Model file for the job. Use its own axes, mm. A direction names the side the tool comes from. Give positions to 0.01 mm unless a question says otherwise; leave off trailing zeros. Write each loop counter-clockwise with the first axis right and the second up, starting at its lowest first coordinate (ties: lowest second). Pieces come first, ordered by that corner, then holes. Notation, with made-up numbers: (58.25, 64) - (62.25, 64) arc R29 ccw to (62.25, 87) - close; hole circle Ø9 at (41.5, 72). An arc over 180 degrees is marked (long way). One line per item, written item: value. Start each with the question number.
(1) Cut at D-D, the plane x = -23. List the corners of the cut face in (y, z).
(2) Cut at A-A, the plane x = 0. List the corners of the cut face in (y, z), and give its area (3 significant figures).
(3) Drop flat-ended pins along their axis: P1, Ø8, axis at y = -27.5, z = 14.5, coming from the -X side; P2, Ø1.5, axis at y = 27.5, z = 11.5, coming from the -X side; P3, Ø8, axis at x = 12, z = 7.5, coming from the -Y side. Give the stop position or say it passes through.
(4) Cut at C-C, the plane y = 63.5. List the corners of the cut face in (x, z), and give its area (3 significant figures).
(5) Cut at B-B, the plane y = 0. List the corners of the cut face in (x, z).
(6) Mould opens along Y. For faces 6 (the face through (-35.2, -72.74, 12.52)), 7 (the face through (25.17, 51.98, 12.52)), 8 (the face through (-19, 3, 25.4)), 9 (the face through (-56.276, 12.977, 12.522)) say: pulls with the +Y half, pulls with the -Y half, needs draft (parallel to the pull), parting line crosses it, or undercut.
(7) Probe L1, parallel to Y at x = 0, z = 10.5; L2, parallel to X at y = 56, z = 14; L3, parallel to X at y = -58, z = 14. List the from-to ranges inside material, lowest first.
(8) 3-axis set-ups, long thin cutter, end or side, ignore diameter. For faces 1 (the face through (-45.39, 53.94, 12.52)), 2 (the face through (70.77, -2, 12.52)), 3 (the face through (17.49, -68.29, 12.52)), 4 (the face through (-42.49, -56.26, 12.52)), 5 (the face through (34.922, -72.876, 12.522)): which of +Z, -Z, +X, -X, +Y, -Y reach the whole face in a straight line?
from build123d import *

# Parameters (mm, degrees)
F0_R     = 19.05
F1_DEPTH = 25.4


with BuildPart() as f1:
    # F0 (on Top) → F1 (new body)
    with BuildSketch(Plane.XY):
        with BuildLine():
            Line((-10.182837, -59.196547), (-9.157953, -57.02169))
            ThreePointArc((-9.157953, -57.02169), (-25.057833, -52.033126), (-38.871462, -42.712418))
            Line((-38.871462, -42.712418), (-39.932829, -44.869706))
            Line((-39.932829, -44.869706), (-45.115972, -67.966514))
            Line((-45.115972, -67.966514), (-35.062492, -72.808015))
            Line((-35.062492, -72.808015), (-25.009012, -77.649516))
            Line((-25.009012, -77.649516), (-10.182837, -59.196547))
        make_face()
        with BuildLine():
            Line((-52.630619, -28.947181), (-50.291243, -28.392466))
            ThreePointArc((-50.291243, -28.392466), (-56.30444, -12.851121), (-57.629873, 3.760176))
            Line((-57.629873, 3.760176), (-59.97826, 3.244939))
            Line((-59.97826, 3.244939), (-81.267709, -7.103341))
            Line((-81.267709, -7.103341), (-78.784705, -17.982095))
            Line((-78.784705, -17.982095), (-76.3017, -28.860849))
            Line((-76.3017, -28.860849), (-52.630619, -28.947181))
        make_face()
        with BuildLine():
            ThreePointArc((-53.554201, 21.616864), (-45.152655, 36.008041), (-32.991815, 47.401281))
            Line((-32.991815, 47.401281), (-34.858838, 48.916078))
            Line((-34.858838, 48.916078), (-56.223203, 59.108793))
            Line((-56.223203, 59.108793), (-63.180428, 50.38471))
            Line((-63.180428, 50.38471), (-70.137652, 41.660627))
            Line((-70.137652, 41.660627), (-55.446471, 23.100003))
            Line((-55.446471, 23.100003), (-53.554201, 21.616864))
        make_face()
        with BuildLine():
            ThreePointArc((32.991815, 47.401281), (45.152655, 36.008041), (53.554201, 21.616864))
            Line((53.554201, 21.616864), (55.446471, 23.100003))
            Line((55.446471, 23.100003), (70.137652, 41.660627))
            Line((70.137652, 41.660627), (63.180428, 50.38471))
            Line((63.180428, 50.38471), (56.223203, 59.108793))
            Line((56.223203, 59.108793), (34.858838, 48.916078))
            Line((34.858838, 48.916078), (32.991815, 47.401281))
        make_face()
        with BuildLine():
            ThreePointArc((0, 57.752413), (8.332046, 57.148213), (16.489754, 55.348254))
            Line((16.489754, 55.348254), (16.51, 57.752413))
            Line((16.51, 57.752413), (11.158521, 80.8108))
            Line((11.158521, 80.8108), (0, 80.8108))
            Line((0, 80.8108), (0, 57.752413))
        make_face()
        with BuildLine():
            ThreePointArc((-16.489754, 55.348254), (-8.332046, 57.148213), (0, 57.752413))
            Line((0, 57.752413), (0, 80.8108))
            Line((0, 80.8108), (-11.158521, 80.8108))
            Line((-11.158521, 80.8108), (-16.51, 57.752413))
            Line((-16.51, 57.752413), (-16.489754, 55.348254))
        make_face()
        with BuildLine():
            ThreePointArc((57.629873, 3.760176), (57.72177, 1.881086), (57.752413, 0))
            ThreePointArc((57.752413, 0), (55.855984, -14.678225), (50.291243, -28.392466))
            Line((50.291243, -28.392466), (52.630619, -28.947181))
            Line((52.630619, -28.947181), (76.3017, -28.860849))
            Line((76.3017, -28.860849), (78.784705, -17.982095))
            Line((78.784705, -17.982095), (81.267709, -7.103341))
            Line((81.267709, -7.103341), (59.97826, 3.244939))
            Line((59.97826, 3.244939), (57.629873, 3.760176))
        make_face()
        with BuildLine():
            Line((39.932829, -44.869706), (38.871462, -42.712418))
            ThreePointArc((38.871462, -42.712418), (25.057833, -52.033126), (9.157953, -57.02169))
            Line((9.157953, -57.02169), (10.182837, -59.196547))
            Line((10.182837, -59.196547), (25.009012, -77.649516))
            Line((25.009012, -77.649516), (35.062492, -72.808015))
            Line((35.062492, -72.808015), (45.115972, -67.966514))
            Line((45.115972, -67.966514), (39.932829, -44.869706))
        make_face()
        with BuildLine():
            ThreePointArc((50.291243, -28.392466), (55.855984, -14.678225), (57.752413, 0))
            ThreePointArc((57.752413, 0), (57.72177, 1.881086), (57.629873, 3.760176))
            ThreePointArc((57.629873, 3.760176), (56.30444, 12.851121), (53.554201, 21.616864))
            ThreePointArc((53.554201, 21.616864), (45.152655, 36.008041), (32.991815, 47.401281))
            ThreePointArc((32.991815, 47.401281), (25.057833, 52.033126), (16.489754, 55.348254))
            ThreePointArc((16.489754, 55.348254), (8.332046, 57.148213), (0, 57.752413))
            ThreePointArc((0, 57.752413), (-8.332046, 57.148213), (-16.489754, 55.348254))
            ThreePointArc((-16.489754, 55.348254), (-25.057833, 52.033126), (-32.991815, 47.401281))
            ThreePointArc((-32.991815, 47.401281), (-45.152655, 36.008041), (-53.554201, 21.616864))
            ThreePointArc((-53.554201, 21.616864), (-56.30444, 12.851121), (-57.629873, 3.760176))
            ThreePointArc((-57.629873, 3.760176), (-56.30444, -12.851121), (-50.291243, -28.392466))
            ThreePointArc((-50.291243, -28.392466), (-45.152655, -36.008041), (-38.871462, -42.712418))
            ThreePointArc((-38.871462, -42.712418), (-25.057833, -52.033126), (-9.157953, -57.02169))
            ThreePointArc((-9.157953, -57.02169), (0, -57.752413), (9.157953, -57.02169))
            ThreePointArc((9.157953, -57.02169), (25.057833, -52.033126), (38.871462, -42.712418))
            ThreePointArc((38.871462, -42.712418), (45.152655, -36.008041), (50.291243, -28.392466))
        make_face()
        Circle(F0_R, mode=Mode.SUBTRACT)
    extrude(amount=F1_DEPTH)


solid = f1.part
Answers follow:
1. outline: (-75.15, 0) - (52.97, 0) - (52.97, 25.4) - (-75.15, 25.4) - close
2. outline: (-57.75, 0) - (-19.05, 0) - (-19.05, 25.4) - (-57.75, 25.4) - close; (19.05, 0) - (80.81, 0) - (80.81, 25.4) - (19.05, 25.4) - close
2. area: 2,550 mm²
3. P1: stops at x = -77.53
3. P2: stops at x = -59.52
3. P3: stops at y = -66.44
4. outline: (-15.18, 0) - (15.18, 0) - (15.18, 25.4) - (-15.18, 25.4) - close
4. area: 771 mm²
5. outline: (-66.65, 0) - (-19.05, 0) - (-19.05, 25.4) - (-66.65, 25.4) - close; (19.05, 0) - (66.65, 0) - (66.65, 25.4) - (19.05, 25.4) - close
6. face 6: pulls with the -Y half
6. face 7: pulls with the +Y half
6. face 8: needs draft
6. face 9: undercut
7. L1: y = -57.75 to -19.05, 19.05 to 80.81
7. L2: x = -58.7 to -49.71, -16.5 to 16.5, 49.71 to 58.7
7. L3: x = -42.88 to -9.62, 9.62 to 42.88
8. face 1: +Z, -Z, +Y
8. face 2: +Z, -Z, +X
8. face 3: +Z, -Z, -Y
8. face 4: +Z, -Z, -X
8. face 5: +Z, -Z, +X, -Y
